```python
from build123d import *

# Parameters (mm, degrees)
BOSS_EXTRUDE1_DEPTH = 10
FILLET1_R           = 1


with BuildPart() as part:
    # Sketch1 → Boss-Extrude1 (new body)
    with BuildSketch(Plane(origin=(0, 0, 0), x_dir=(1, 0, 0), z_dir=(0, 1, 0))):
        Polygon((33.044354839, 55), (44.567912368, 45.070610508), (36.814516129, 32.822580645), (50, 15.302419355), (36.814516129, 0), (0, 0), (0, 55), align=None)
        Polygon((8.987912628, 48.788514125), (8.987912628, 4.213709677), (28.947590047, 4.213709677), (38.589466872, 15.403594249), (29.007221014, 28.135966803), (13.109814871, 28.135966803), (18.704963548, 35.611652929), (29.007221014, 35.611652929), (33.844976201, 43.25384845), (27.421717413, 48.788514125), align=None, mode=Mode.SUBTRACT)
    extrude(amount=BOSS_EXTRUDE1_DEPTH)

    # Fillet1
    fillet1_edges = [part.edges().sort_by_distance(p)[0] for p in [
        (0, 5, -55),
        (33.044354839, 5, -55),
        (44.567912368, 5, -45.070610508),
        (36.814516129, 5, -32.822580645),
        (50, 5, -15.302419355),
        (36.814516129, 5, 0),
        (0, 5, 0),
        (8.987912628, 5, -4.213709677),
        (13.109814871, 5, -28.135966803),
        (18.704963548, 5, -35.611652929),
    ]]
    fillet(fillet1_edges, radius=FILLET1_R)


solid = part.part
```
Geometry: final body of the model. Coordinates: model frame, mm. A direction names the side the tool comes from. Coordinates: 2 decimals unless noted, no trailing zeros. Order: outer loops, then holes, each group sorted by start corner. A loop starts at its lowest first (then second) coordinate and runs counter-clockwise, first axis right, second up. Notation, with made-up numbers: (77, -1.75) - (100, -1.75) arc R13 cw to (100, 7.25) - close; hole circle Ø6 at (81.5, -20.75). An arc over 180 degrees is marked (long way). Write each question's results on one line, items separated by ' | '.
(1) First-contact query: pin 1 Ø3 at (x, y) = (41, 3) entering from -Z; pin 2 Ø6 at (x, z) = (42.5, -41) entering from -Y; pin 3 Ø5 at (y, z) = (5, -30) entering from +X; pin 4 Ø8 at (x, z) = (18.5, -41.5) entering from -Y. Flat tips, straight axial feed; report the tip coordinate or a pass-through.
Values found:
pin 1: stops at z = -49.44 | pin 2: stops at y = 0 | pin 3: stops at x = 40.82 | pin 4: passes through
(2) Mould query, pull axis X, two halves, no side actions, for faces 4 (the face through (20, 10, -34)), 5 (the face through (19, 5, -4.214)), 6 (the face through (18, 5, -48.789)), 7 (the face through (49.716, 5.07, -15.321)). Classes: +X half, -X half, draft (parallel to the pull), parting line (faces both ways), or undercut.
Values found:
face 4: draft | face 5: undercut | face 6: undercut | face 7: +X half
(3) Set-up query: faces 1 (the face through (8.988, 5, -27)), 2 (the face through (40.694, 4.93, -38.951)), 3 (the face through (38.5, 4.9, -50.3)). Return all of +Z, -Z, +X, -X, +Y, -Y with unobstructed straight access to the full face (end or side cutting, diameter ignored); none if empty.
Values found:
face 1: +Y, -Y | face 2: +X, +Y, -Y | face 3: -Z, +X, +Y, -Y
(4) Line query: line 1 (Z direction, x = 21.5, y = 8.25); line 2 (Z direction, x = 14, y = 5); line 3 (Z direction, x = 28.5, y = 9.25). Output: solid intervals per line, ascending. Write a range as [from, to].
Values found:
line 1: z = [-55, -48.79], [-35.61, -28.14], [-4.21, 0] | line 2: z = [-55, -48.79], [-4.21, 0] | line 3: z = [-55, -47.86], [-35.61, -28.14], [-4.21, 0]
(5) Section query B-B, the plane x = 12. Return the cut outline in (y, z).
Values found:
outline: (0, -55) - (10, -55) - (10, -48.79) - (0, -48.79) - close; (0, -4.21) - (10, -4.21) - (10, 0) - (0, 0) - close
(6) Section query C-C, the plane y = 7. Return the cut outline in (x, z), plus the area to 3 significant figures.
Values found:
outline: (0, -54) arc R1 ccw to (1, -55) - (32.67, -55) arc R1 ccw to (33.33, -54.76) - (43.91, -45.63) arc R1 ccw to (44.11, -44.34) - (37.18, -33.41) arc R1 cw to (37.23, -32.27) - (49.52, -15.95) arc R1 ccw to (49.47, -14.69) - (37.11, -0.35) arc R1 ccw to (36.36, 0) - (1, 0) arc R1 ccw to (0, -1) - close; hole (8.99, -48.79) - (27.42, -48.79) - (33.84, -43.25) - (29.01, -35.61) - (19.21, -35.61) arc R1 cw to (18.4, -35.21) - (14.31, -29.74) arc R1 cw to (15.11, -28.14) - (29.01, -28.14) - (38.59, -15.4) - (28.95, -4.21) - (9.99, -4.21) arc R1 ccw to (8.99, -5.21) - close | area: 1,370 mm²
(7) Section query D-D, the plane z = -21. Return the cut outline in (x, y).
Values found:
outline: (0, 0) - (8.99, 0) - (8.99, 10) - (0, 10) - close; (34.38, 0) - (45.71, 0) - (45.71, 10) - (34.38, 10) - close
(8) Section query A-A, the plane x = 20. Return the cut outline in (y, z), plus the area to 3 significant figures.
Values found:
outline: (0, -55) - (10, -55) - (10, -48.79) - (0, -48.79) - close; (0, -35.61) - (10, -35.61) - (10, -28.14) - (0, -28.14) - close; (0, -4.21) - (10, -4.21) - (10, 0) - (0, 0) - close | area: 179 mm²
